from build123d import *

# Parameters (mm, degrees)
SKETCH1_R           = 50.8
SKETCH1_R_2         = 9.525
BOSS_EXTRUDE1_DEPTH = 3.175
SKETCH2_R           = 3.175
BOSS_EXTRUDE2_DEPTH = 44.45


with BuildPart() as part:
    # Sketch1 → Boss-Extrude1 (new body)
    with BuildSketch(Plane(origin=(0, 0, 0), x_dir=(1, 0, 0), z_dir=(0, 1, 0))):
        with Locations(Location((0, 0, 0), (0, 0, 270))):
            Circle(SKETCH1_R)
        with Locations(Location((0, 0, 0), (0, 0, 270))):
            Circle(SKETCH1_R_2, mode=Mode.SUBTRACT)
    extrude(amount=BOSS_EXTRUDE1_DEPTH)

    # Sketch2 → Boss-Extrude2 (add)
    with BuildSketch(Plane(origin=(0, 3.175, 0), x_dir=(1, 0, 0), z_dir=(0, 1, 0))):
        with Locations(Location((-9.214642662, 43.945595463, 0), (0, 0, 270))):
            Circle(SKETCH2_R)
        with Locations(Location((43.945595463, 9.214642662, 0), (0, 0, 270))):
            Circle(SKETCH2_R)
        with Locations(Location((9.214642662, -43.945595463, 0), (0, 0, 270))):
            Circle(SKETCH2_R)
        with Locations(Location((-43.945595463, -9.214642662, 0), (0, 0, 270))):
            Circle(SKETCH2_R)
    extrude(amount=BOSS_EXTRUDE2_DEPTH)


solid = part.part
CAD build for the part. Positions are in the model's coordinates, mm. A direction names the side the tool comes from. Round coordinates to 2 decimals unless told otherwise and drop trailing zeros. Write each loop counter-clockwise with the first axis right and the second up, starting at its lowest first coordinate (ties: lowest second). Pieces come first, ordered by that corner, then holes. Notation, with made-up numbers: M 1,59 L 34,59 A34 ccw 34,97 Z; hole C 69.5,35 d4. An arc over 180 degrees is marked long. Use a Markdown table: item, result. Add a question column.
1. 3-axis set-ups, long thin cutter, end or side, ignore diameter. For faces 1 (the face through (8, 25.09, 46.88)), 2 (the face through (9, 47.625, 44)): which of +Z, -Z, +X, -X, +Y, -Y reach the whole face in a straight line?
2. Slice it at A-A on z = 0. Give the cut face in (x, y) (3 decimals), then the cut area to 3 significant figures.
3. Flat gauge pins, fed straight in: P1, Ø5, axis at x = 0.5, z = -26.5, coming from the -Y side; P2, Ø4, axis at x = -6, y = 19, coming from the -Z side; P3, Ø5, axis at y = 29.5, z = 12, coming from the +X side; P4, Ø11.5, axis at x = 0, z = 0, coming from the +Y side. Where does each tip first touch, or does it go through?
4. Drill centre lines: probe 1 along X at (y, z) = (1, 0) (3 decimals); probe 2 along Y at (x, z) = (-2, -42) (3 decimals); probe 3 along X at (y, z) = (3, 17). Where is each one in solid material? Low to high.
5. Slice it at C-C on y = 22. Give the cut face in (x, z) (3 decimals), then the cut area to 3 significant figures.
6. Pull direction Z, two halves, no side cores. Call faces 3 (the face through (-40.798, 25.089, 8.801)), 4 (the face through (-9, 47.625, -44)), 5 (the face through (-5.796, 1.565, -7.559)): released by +Z, released by -Z, zero draft, split by the parting line, or undercut.
7. Slice it at D-D on z = -26.5. Give the cut face in (x, y) (3 decimals), then the cut area to 3 significant figures.
8. Slice it at B-B on x = 8. Give the cut face in (y, z) (3 decimals).
Reply:
| question | item | result |
|---|---|---|
| 1 | face 1 | +Y |
| 1 | face 2 | +Z, -Z, +X, -X, +Y |
| 2 | outline | M -50.8,0 L -9.525,0 L -9.525,3.175 L -50.8,3.175 Z; M 9.525,0 L 50.8,0 L 50.8,3.175 L 9.525,3.175 Z |
| 2 | area | 262 mm^2 |
| 3 | P1 | stops at y = 0 |
| 3 | P2 | stops at z = -46.88 |
| 3 | P3 | stops at x = -40.78 |
| 3 | P4 | passes through |
| 4 | probe 1 | x = -50.8 to -9.525, 9.525 to 50.8 |
| 4 | probe 2 | y = 0 to 3.175 |
| 4 | probe 3 | x = -47.87 to 47.87 |
| 5 | outline | C -43.946,9.215 d6.35; C -9.215,-43.946 d6.35; C 9.215,43.946 d6.35; C 43.946,-9.215 d6.35 |
| 5 | area | 127 mm^2 |
| 6 | face 3 | split by the parting line |
| 6 | face 4 | zero draft |
| 6 | face 5 | undercut |
| 7 | outline | M -43.34,0 L 43.34,0 L 43.34,3.175 L -43.34,3.175 Z |
| 7 | area | 275 mm^2 |
| 8 | outline | M 0,-50.166 L 3.175,-50.166 L 3.175,-5.17 L 0,-5.17 Z; M 0,5.17 L 3.175,5.17 L 3.175,41.012 L 47.625,41.012 L 47.625,46.879 L 3.175,46.879 L 3.175,50.166 L 0,50.166 Z |
